from build123d import *

# Parameters (mm, degrees)
F0_R     = 7.125
F1_DEPTH = 24.45
F2_R     = 2.65
F3_DEPTH = 1.55
F4_R     = 0.5
F5_R     = 1


with BuildPart() as f1:
    # F0 (on Top) → F1 (new body, symmetric)
    with BuildSketch(Plane.XY):
        Circle(F0_R)
    extrude(amount=F1_DEPTH, both=True)

    # F2 (on face) → F3 (join)
    with BuildSketch(Plane.XY.offset(24.45)):
        Circle(F2_R)
    extrude(amount=F3_DEPTH)

    # F4
    f4_edges = [f1.edges().sort_by_distance(p)[0] for p in [
        (-2.65, 0, 26),
    ]]
    fillet(f4_edges, radius=F4_R)

    # F5
    f5_edges = [f1.edges().sort_by_distance(p)[0] for p in [
        (-7.125, 0, 24.45),
        (-7.125, 0, -24.45),
    ]]
    fillet(f5_edges, radius=F5_R)


solid = f1.part
Check sheet for the modelled part. Datum: model origin and axes. Units: mm. A direction names the side the tool comes from. Round coordinates to 2 decimals unless told otherwise and drop trailing zeros. Loops run counter-clockwise (first coordinate to the right, second up) from the corner with the lowest first, then second, coordinate; pieces in that order, holes last.
1. Gauge pin test, flat ends, axial feed: pin 1 Ø6 at (x, z) = (-5, -0.5) entering from +Y; pin 2 Ø4 at (y, z) = (2, -10.5) entering from +X (3 decimals); pin 3 Ø1 at (x, y) = (3.5, -0.5) entering from +Z. Record the tip position at first contact, or that the pin passes through.
2. Sectioned sample at C-C on z = -4. Record the boundary of the cut face in (x, y) (3 decimals).
3. Scan lines: probe 1 along Z at (x, y) = (4.5, -4); probe 2 along X at (y, z) = (-0.25, -19.5); probe 3 along Y at (x, z) = (1.75, 1.5). Record each from-to range of solid material in increasing order.
4. Set-up check for faces 1 (the cylindrical face through (2.45, -1.01, 24.97)), 2 (the flat face through (0, 0, 26)): record each of +Z, -Z, +X, -X, +Y, -Y from which the full face is reachable in a straight line by a thin tool's end or side.
5. Sectioned sample at A-A on x = 0. Record the boundary of the cut face in (y, z) (3 decimals).
Recorded:
1. pin 1: stops at y = 6.84
1. pin 2: stops at x = 7.125
1. pin 3: stops at z = 24.45
2. outline: circle Ø14.25 at (0, 0)
3. probe 1: z = -24.45 to 24.45
3. probe 2: x = -7.12 to 7.12
3. probe 3: y = -6.91 to 6.91
4. face 1: +Z
4. face 2: +Z, +X, -X, +Y, -Y
5. outline: (-7.125, -23.45) arc R1 ccw to (-6.125, -24.45) - (6.125, -24.45) arc R1 ccw to (7.125, -23.45) - (7.125, 23.45) arc R1 ccw to (6.125, 24.45) - (2.65, 24.45) - (2.65, 25.5) arc R0.5 ccw to (2.15, 26) - (-2.15, 26) arc R0.5 ccw to (-2.65, 25.5) - (-2.65, 24.45) - (-6.125, 24.45) arc R1 ccw to (-7.125, 23.45) - close
